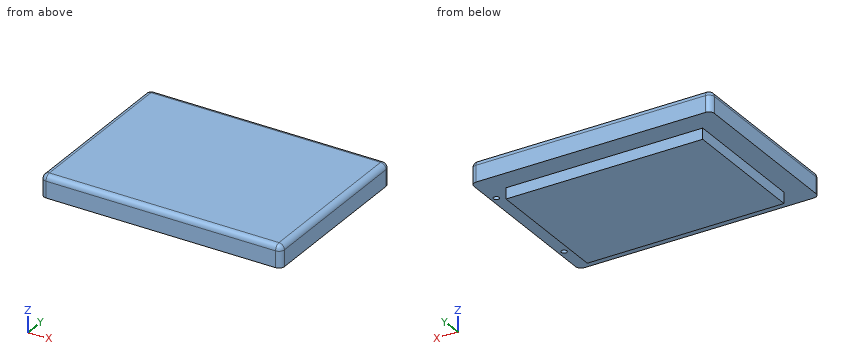
from build123d import *

# Parameters (mm, degrees)
SKETCH_1_W          = 440
SKETCH_1_H          = 320
EXTRUDE_1_DEPTH     = 40
FILLET_1_R          = 10
SKETCH_3_W          = 360
SKETCH_3_H          = 240
EXTRUDE_2_DEPTH     = 20
SKETCH_4_R          = 5
CUT_EXTRUDE_1_DEPTH = 10


with BuildPart() as part:
    # 草图1 → 凸台-拉伸1 (new body)
    with BuildSketch(Plane.XY):
        with Locations((220, -160)):
            Rectangle(SKETCH_1_W, SKETCH_1_H)
    extrude(amount=EXTRUDE_1_DEPTH)

    # 圆角1
    fillet_1_edges = [part.edges().sort_by_distance(p)[0] for p in [
        (440, -160, 40),
        (220, 0, 40),
        (0, -160, 40),
        (0, 0, 20),
        (440, 0, 20),
        (440, -320, 20),
        (0, -320, 20),
        (220, -320, 40),
    ]]
    fillet(fillet_1_edges, radius=FILLET_1_R)

    # 草图3 → 凸台-拉伸2 (add)
    with BuildSketch(Plane(origin=(0, 0, 0), x_dir=(-1, 0, 0), z_dir=(0, 0, -1))):
        with Locations((-220, -160)):
            Rectangle(SKETCH_3_W, SKETCH_3_H)
    extrude(amount=EXTRUDE_2_DEPTH)

    # 草图4 → 切除-拉伸1 (cut)
    with BuildSketch(Plane(origin=(0, 0, 0), x_dir=(-1, 0, 0), z_dir=(0, 0, -1))):
        with Locations((-430, -60)):
            Circle(SKETCH_4_R)
        with Locations((-430, -260)):
            Circle(SKETCH_4_R)
    extrude(amount=-CUT_EXTRUDE_1_DEPTH, mode=Mode.SUBTRACT)


solid = part.part
Can you work these out from the model? Positions are in its coordinate system, mm. Coordinates: 2 decimals unless noted, no trailing zeros. Loops run counter-clockwise (first coordinate to the right, second up) from the corner with the lowest first, then second, coordinate; pieces in that order, holes last. Notation, with made-up numbers: (37.25, 75.25) - (71.25, 75.25) arc R19 ccw to (71.25, 98.25) - close; hole circle Ø7 at (36, 70.25). An arc over 180 degrees is marked (long way). Answer as a JSON object with one key per item and string values. Group by question number.
Item 1: If I drill on L1, parallel to Y at x = 430, z = 7; L2, parallel to X at y = -260, z = 4; L3, parallel to Z at x = 422.5, y = -251.5, over which ranges is the centre line in solid material (lowest first)? Write a range as from..to.
Item 2: For pin 1 (3 mm diameter, centred on y = -250, z = 33, fed in from +X); pin 2 (6 mm diameter, centred on x = 199.5, z = 30.5, fed in from +Y); pin 3 (10 mm diameter, centred on x = 213.5, z = -14, fed in from +Y); pin 4 (10 mm diameter, centred on y = -108.5, z = -13.5, fed in from +X), each with a flat end and sliding along its axis, tell me the tip position at first contact or that it passes through.
Item 3: If we section it at C-C (y = -178): List the corners of the cut face in (x, z) for me.
Item 4: If we section it at A-A (y = -260): List the corners of the cut face in (x, z) for me.
Item 5: If we section it at B-B (x = 160.5): List the corners of the cut face in (y, z) for me.
Returned:
{
 "1": {"L1": "y = -320..-265, -255..-65, -55..0", "L2": "x = 0..425, 435..440", "L3": "z = 0..40"},
 "2": {"pin 1": "stops at x = 439.89", "pin 2": "stops at y = 0", "pin 3": "stops at y = -40", "pin 4": "stops at x = 400"},
 "3": {"outline": "(0, 0) - (40, 0) - (40, -20) - (400, -20) - (400, 0) - (440, 0) - (440, 30) arc R10 ccw to (430, 40) - (10, 40) arc R10 ccw to (0, 30) - close"},
 "4": {"outline": "(0, 0) - (40, 0) - (40, -20) - (400, -20) - (400, 0) - (425, 0) - (425, 10) - (435, 10) - (435, 0) - (440, 0) - (440, 30) arc R10 ccw to (430, 40) - (10, 40) arc R10 ccw to (0, 30) - close"},
 "5": {"outline": "(-320, 0) - (-280, 0) - (-280, -20) - (-40, -20) - (-40, 0) - (0, 0) - (0, 30) arc R10 ccw to (-10, 40) - (-310, 40) arc R10 ccw to (-320, 30) - close"}
}
